from build123d import *

# Parameters (mm, degrees)
SKETCH_1_R          = 3
SKETCH_1_R_2        = 1.55
EXTRUDE_1_DEPTH     = 30
CUT_EXTRUDE_1_DEPTH = 37.5
SKETCH_4_W          = 30
SKETCH_4_H          = 30
CUT_EXTRUDE_3_DEPTH = 12
EXTRUDE_2_DEPTH     = 55
SKETCH_6_R          = 2.3
SKETCH_6_R_2        = 5
SKETCH_6_R_3        = 6
SKETCH_6_R_4        = 4
CUT_EXTRUDE_4_DEPTH = 25.5
FILLET_2_R          = 2
CUT_EXTRUDE_5_DEPTH = 25.5


with BuildPart() as part:
    # 草图1 → 凸台-拉伸1 (new body)
    with BuildSketch(Plane.XY):
        Polygon((15, 0), (15, 12.5), (0, 12.5), (-15, 12.5), (-15, -24), (15, -24), align=None)
        Circle(SKETCH_1_R, mode=Mode.SUBTRACT)
        with Locations((-5, 5)):
            Circle(SKETCH_1_R_2, mode=Mode.SUBTRACT)
        with Locations((-5, -5)):
            Circle(SKETCH_1_R_2, mode=Mode.SUBTRACT)
        with Locations((5, -5)):
            Circle(SKETCH_1_R_2, mode=Mode.SUBTRACT)
        with Locations((5, 5)):
            Circle(SKETCH_1_R_2, mode=Mode.SUBTRACT)
    extrude(amount=EXTRUDE_1_DEPTH)

    # 草图2 → 切除-拉伸1 (cut, through all)
    with BuildSketch(Plane(origin=(0, 12.5, 0), x_dir=(1, 0, 0), z_dir=(0, 1, 0))):
        Polygon((-11.4, -15), (-11.4, -3.6), (0, -3.6), (11.4, -3.6), (11.4, -26.4), (0, -26.4), (-11.4, -26.4), align=None)
    extrude(amount=-CUT_EXTRUDE_1_DEPTH, mode=Mode.SUBTRACT)

    # 草图4 → 切除-拉伸3 (cut)
    with BuildSketch(Plane.XZ.offset(24)):
        with Locations((0, 15)):
            Rectangle(SKETCH_4_W, SKETCH_4_H)
    extrude(amount=-CUT_EXTRUDE_3_DEPTH, mode=Mode.SUBTRACT)

    # 草图5 → 凸台-拉伸2 (add)
    with BuildSketch(Plane.ZY.offset(15)):
        Polygon((30, -12), (30, 11.596689914), (30, 12.5), (0, 12.5), (0, -12), align=None)
    extrude(amount=EXTRUDE_2_DEPTH)

    # 草图6 → 切除-拉伸4 (cut, through all)
    with BuildSketch(Plane(origin=(0, 12.5, 0), x_dir=(1, 0, 0), z_dir=(0, 1, 0))):
        Polygon((-70, -15), (-11.4, 0), (-70, 0), align=None)
        Polygon((-11.4, -30), (-70, -15), (-70, -30), align=None)
        with Locations((-56.4, -15)):
            Circle(SKETCH_6_R)
        with Locations((-33.9, -15)):
            Circle(SKETCH_6_R_2)
        with Locations((-22.125549979, -15)):
            Circle(SKETCH_6_R_3)
        with Locations((-46.110471912, -15)):
            Circle(SKETCH_6_R_4)
    extrude(amount=-CUT_EXTRUDE_4_DEPTH, mode=Mode.SUBTRACT)

    # 圆角2
    fillet_2_edges = [part.edges().sort_by_distance(p)[0] for p in [
        (-70, 0.25, 15),
    ]]
    fillet(fillet_2_edges, radius=FILLET_2_R)

    # 草图7 → 切除-拉伸5 (cut, through all)
    with BuildSketch(Plane(origin=(0, 12.5, 0), x_dir=(1, 0, 0), z_dir=(0, 1, 0))):
        Polygon((-11.4, -3.6), (-11.4, 0), (-66.954884603, 0), (-66.4, -30), (-11.4, -30), align=None)
    extrude(amount=-CUT_EXTRUDE_5_DEPTH, mode=Mode.SUBTRACT)


solid = part.part
Could you check a few things on this model? Use its own coordinates, in mm. A direction names the side the tool comes from. Coordinates: 2 decimals unless noted, no trailing zeros. Loops run counter-clockwise (first coordinate to the right, second up) from the corner with the lowest first, then second, coordinate; pieces in that order, holes last. Notation, with made-up numbers: (-3, 19) -> (48, 19) arc R20 ccw to (48, 43) -> close; hole circle Ø2 at (83, -5.75). An arc over 180 degrees is marked (long way). Answer in a Markdown table with one row per item.
(1) If I drill on probe 1 along X at (y, z) = (-5, 28.9); probe 2 along Y at (x, z) = (-5, 28.15); probe 3 along Z at (x, y) = (7.25, 7.5), over which ranges is the centre line in solid material (lowest first)?
Results found:
| item | result |
|---|---|
| probe 1 | x = -11.4 to -6.55, -3.45 to 3.45, 6.55 to 15 |
| probe 2 | y = -12 to -6.55, -3.45 to 3.45, 6.55 to 12.5 |
| probe 3 | z = 0 to 3.6, 26.4 to 30 |
(2) Imagine slicing it at A-A (x = -5). List the corners of the cut face in (y, z) for me, plus the area to 3 significant figures.
Results found:
| item | result |
|---|---|
| outline | (-12, 0) -> (-6.55, 0) -> (-6.55, 3.6) -> (-12, 3.6) -> close; (-12, 26.4) -> (-6.55, 26.4) -> (-6.55, 30) -> (-12, 30) -> close; (-3.45, 0) -> (3.45, 0) -> (3.45, 3.6) -> (-3.45, 3.6) -> close; (-3.45, 26.4) -> (3.45, 26.4) -> (3.45, 30) -> (-3.45, 30) -> close; (6.55, 0) -> (12.5, 0) -> (12.5, 3.6) -> (6.55, 3.6) -> close; (6.55, 26.4) -> (12.5, 26.4) -> (12.5, 30) -> (6.55, 30) -> close |
| area | 132 mm^2 |
(3) Will these pins go through, and if not, where does the flat tip stop? pin 1 Ø3 at (x, y) = (5, 5) entering from -Z; pin 2 Ø7 at (y, z) = (-0.5, 10.5) entering from -X.
Results found:
| item | result |
|---|---|
| pin 1 | passes through |
| pin 2 | stops at x = 11.4 |
(4) Imagine slicing it at C-C (y = 0). List the corners of the cut face in (x, z) for me.
Results found:
| item | result |
|---|---|
| outline | (-11.4, 0) -> (-3, 0) -> (-3, 3.6) -> (-11.4, 3.6) -> close; (-11.4, 26.4) -> (-3, 26.4) -> (-3, 30) -> (-11.4, 30) -> close; (3, 0) -> (15, 0) -> (15, 30) -> (3, 30) -> (3, 26.4) -> (11.4, 26.4) -> (11.4, 3.6) -> (3, 3.6) -> close |
(5) Imagine slicing it at B-B (y = 5). List the corners of the cut face in (x, z) for me, plus the area to 3 significant figures.
Results found:
| item | result |
|---|---|
| outline | (-11.4, 0) -> (-6.55, 0) -> (-6.55, 3.6) -> (-11.4, 3.6) -> close; (-11.4, 26.4) -> (-6.55, 26.4) -> (-6.55, 30) -> (-11.4, 30) -> close; (-3.45, 0) -> (3.45, 0) -> (3.45, 3.6) -> (-3.45, 3.6) -> close; (-3.45, 26.4) -> (3.45, 26.4) -> (3.45, 30) -> (-3.45, 30) -> close; (6.55, 0) -> (15, 0) -> (15, 30) -> (6.55, 30) -> (6.55, 26.4) -> (11.4, 26.4) -> (11.4, 3.6) -> (6.55, 3.6) -> close |
| area | 228 mm^2 |
(6) Thinking about a two-plate mould opening in Y: for faces 3 (the face through (15, 0, 15)), 4 (the face through (3.45, -4.93, 28.17)), 5 (the face through (-6.55, 5.07, 1.77)), 6 (the face through (12, 12.5, 15)), which applies, released by +Y, released by -Y, zero draft, split by the parting line, or undercut?
Results found:
| item | result |
|---|---|
| face 3 | zero draft |
| face 4 | undercut |
| face 5 | undercut |
| face 6 | released by +Y |
(7) Imagine slicing it at D-D (x = 8.25). List the corners of the cut face in (y, z) for me, plus the area to 3 significant figures.
Results found:
| item | result |
|---|---|
| outline | (-12, 0) -> (12.5, 0) -> (12.5, 3.6) -> (-12, 3.6) -> close; (-12, 26.4) -> (12.5, 26.4) -> (12.5, 30) -> (-12, 30) -> close |
| area | 176 mm^2 |
(8) For faces 1 (the face through (3.45, 5.07, 28.17)), 2 (the face through (3, 3, 3.6)), which set-ups out of +Z, -Z, +X, -X, +Y, -Y let a thin tool reach every point of the face, with its end or its side?
Results found:
| item | result |
|---|---|
| face 1 | +Z, -Z |
| face 2 | -X, +Y, -Y |
